```python
from build123d import *

# Parameters (mm, degrees)
SKETCH1_R           = 9.5
SKETCH1_R_2         = 1.75
SKETCH1_R_3         = 2.6
SKETCH1_R_4         = 3.7
SKETCH1_R_5         = 1.6
SKETCH1_R_6         = 1.55
BOSS_EXTRUDE1_DEPTH = 3.175
FILLET1_R           = 5
FILLET2_R           = 2
BOSS_EXTRUDE2_DEPTH = 3.175
FILLET3_R           = 2
FILLET4_R           = 2
BOSS_EXTRUDE3_START = -3.175
SKETCH4_R           = 2.6
BOSS_EXTRUDE3_DEPTH = 3.175
FILLET5_R           = 5


with BuildPart() as part:
    # Sketch1 → Boss-Extrude1 (new body)
    with BuildSketch(Plane(origin=(0, 0, 0), x_dir=(1, 0, 0), z_dir=(0, 1, 0))):
        with BuildLine():
            Line((-20, -12.068401935), (-7.259795863, 5.319338683))
            ThreePointArc((-7.259795863, 5.319338683), (0, 9), (7.259795863, 5.319338683))
            Line((7.259795863, 5.319338683), (20, -12.068401935))
            Line((20, -12.068401935), (20, -27.9))
            Line((20, -27.9), (31.6, -27.9))
            Line((31.6, -27.9), (31.6, -42.165352614))
            ThreePointArc((31.6, -42.165352614), (51.458612907, -58.2971553), (34, -77))
            Line((34, -77), (23.797619048, -77))
            Line((23.797619048, -77), (20, -93.5))
            Line((20, -93.5), (-20, -93.5))
            Line((-20, -93.5), (-31.6, -43.1))
            Line((-31.6, -43.1), (-31.6, -27.9))
            Line((-31.6, -27.9), (-20, -27.9))
            Line((-20, -27.9), (-20, -12.068401935))
        make_face()
        with Locations(Location((34, -59.5, 0), (0, 0, 270))):
            Circle(SKETCH1_R, mode=Mode.SUBTRACT)
        with Locations(Location((28.294653467, -47.264844875, 0), (0, 0, 270))):
            Circle(SKETCH1_R_2, mode=Mode.SUBTRACT)
        with Locations(Location((39.705346533, -71.735155125, 0), (0, 0, 270))):
            Circle(SKETCH1_R_2, mode=Mode.SUBTRACT)
        with Locations(Location((-24, -35.5, 0), (0, 0, 270))):
            Circle(SKETCH1_R_3, mode=Mode.SUBTRACT)
        with Locations(Location((24, -35.5, 0), (0, 0, 270))):
            Circle(SKETCH1_R_3, mode=Mode.SUBTRACT)
        with Locations(Location((0, 0, 0), (0, 0, 270))):
            Circle(SKETCH1_R_4, mode=Mode.SUBTRACT)
        with Locations(Location((-12.5, -39.3, 0), (0, 0, 270))):
            Circle(SKETCH1_R_5, mode=Mode.SUBTRACT)
        with Locations(Location((-6.75, -19.3, 0), (0, 0, 270))):
            Circle(SKETCH1_R_6, mode=Mode.SUBTRACT)
        with Locations(Location((6.75, -19.3, 0), (0, 0, 270))):
            Circle(SKETCH1_R_6, mode=Mode.SUBTRACT)
        with Locations(Location((7.5, -39.3, 0), (0, 0, 90))):
            Circle(SKETCH1_R_5, mode=Mode.SUBTRACT)
        with Locations(Location((7.5, -88.2, 0), (0, 0, 270))):
            Circle(SKETCH1_R_5, mode=Mode.SUBTRACT)
        with Locations(Location((-12.5, -88.2, 0), (0, 0, 90))):
            Circle(SKETCH1_R_5, mode=Mode.SUBTRACT)
        with BuildLine():
            Line((0, -53.5), (-1.291796068, -53.5))
            ThreePointArc((-1.291796068, -53.5), (-17, -59.5), (-1.291796068, -65.5))
            Line((-1.291796068, -65.5), (0, -65.5))
            ThreePointArc((0, -65.5), (6, -59.5), (0, -53.5))
        make_face(mode=Mode.SUBTRACT)
    extrude(amount=BOSS_EXTRUDE1_DEPTH)

    # Fillet1
    fillet1_edges = [part.edges().sort_by_distance(p)[0] for p in [
        (-31.6, 1.5875, 43.1),
        (-31.6, 1.5875, 27.9),
        (-20, 1.5875, 27.9),
        (-20, 1.5875, 12.068401935),
        (20, 1.5875, 12.068401935),
        (20, 1.5875, 27.9),
        (31.6, 1.5875, 27.9),
        (31.6, 1.5875, 42.165352614),
        (23.797619048, 1.5875, 77),
    ]]
    fillet(fillet1_edges, radius=FILLET1_R)

    # Fillet2
    fillet2_edges = [part.edges().sort_by_distance(p)[0] for p in [
        (-20, 1.5875, 93.5),
        (20, 1.5875, 93.5),
    ]]
    fillet(fillet2_edges, radius=FILLET2_R)

    # Sketch3 → Boss-Extrude2 (add)
    with BuildSketch(Plane(origin=(0, 3.175, 0), x_dir=(1, 0, 0), z_dir=(0, 1, 0))):
        Polygon((21.631006471, -86.413558093), (31.631006471, -86.413558093), (31.631006471, -81), (37.631006471, -81), (37.631006471, -92.413558093), (20.25005409, -92.413558093), align=None)
    extrude(amount=-BOSS_EXTRUDE2_DEPTH)

    # Fillet3
    fillet3_edges = [part.edges().sort_by_distance(p)[0] for p in [
        (21.631006471, 1.5875, 86.413558093),
        (31.631006471, 1.5875, 86.413558093),
        (31.631006471, 1.5875, 81),
        (37.631006471, 1.5875, 81),
        (37.631006471, 1.5875, 92.413558093),
    ]]
    fillet(fillet3_edges, radius=FILLET3_R)

    # Fillet4
    # the kernel refuses this fillet: 2 mm, written as the material it adds along each edge
    with BuildSketch(Plane(origin=(20.357070738, 0, 91.948589209), x_dir=(-0.22429460454884337, 0, 0.974521385281143), z_dir=(0, 1, 0))) as fillet4_piece_1:
        with BuildLine():
            CenterArc((1.551860901, 1.686696047), FILLET4_R, 237.495369906, 9.676681216)
            ThreePointArc((0.77593045, -0.156651976), (0.395792845, -0.039554126), (0, 0))
            Line((0, 0), (0.477125378, 0))
        make_face()
    extrude(amount=3.175)
    # the kernel refuses this fillet: 2 mm, written as the material it adds along each edge
    with BuildSketch(Plane(origin=(20.25005409, 3.175, 92.413558093), x_dir=(1, 0, 0), z_dir=(0, -1, 0))) as fillet4_2_piece_1:
        with BuildLine():
            CenterArc((0.898626945, 2), FILLET4_R, 226.75155148, 43.24844852)
            Line((-0.471699589, 0.543220953), (-0.608732242, 0.397543049))
            ThreePointArc((-0.608732242, 0.397543049), (-0.381915572, 0.139094357), (-0.140266399, -0.142566957))
            Line((-0.140266399, -0.142566957), (0, -0.2))
            Line((0, -0.2), (0.898626945, -0.2))
            Line((0.898626945, -0.2), (0.898626945, 0))
        make_face()
    extrude(amount=3.175)

    # Sketch4 → Boss-Extrude3 (add)
    with BuildSketch(Plane(origin=(0, 3.175, 0), x_dir=(1, 0, 0), z_dir=(0, 1, 0)).offset(BOSS_EXTRUDE3_START)):
        with BuildLine():
            Line((13.146507893, -2.714804316), (7.259795863, 5.319338683))
            ThreePointArc((7.259795863, 5.319338683), (0, 9), (-7.259795863, 5.319338683))
            Line((-7.259795863, 5.319338683), (-13.146507893, -2.714804316))
            Line((-13.146507893, -2.714804316), (-20, 2.306830778))
            Line((-20, 2.306830778), (-20, 25))
            Line((-20, 25), (20, 25))
            Line((20, 25), (20, 2.306830778))
            Line((20, 2.306830778), (13.146507893, -2.714804316))
        make_face()
        with Locations(Location((-15, 20, 0), (0, 0, 270))):
            Circle(SKETCH4_R, mode=Mode.SUBTRACT)
        with Locations(Location((15, 20, 0), (0, 0, 270))):
            Circle(SKETCH4_R, mode=Mode.SUBTRACT)
    extrude(amount=BOSS_EXTRUDE3_DEPTH)

    # Fillet5
    fillet5_edges = [part.edges().sort_by_distance(p)[0] for p in [
        (13.146507893, 1.5875, 2.714804316),
        (20, 1.5875, -2.306830778),
        (20, 1.5875, -25),
        (-20, 1.5875, -25),
        (-20, 1.5875, -2.306830778),
        (-13.146507893, 1.5875, 2.714804316),
    ]]
    fillet(fillet5_edges, radius=FILLET5_R)


solid = part.part
```
Geometry: final body of the model. Coordinates: model frame, mm. A direction names the side the tool comes from. Round coordinates to 2 decimals unless told otherwise and drop trailing zeros. Order: outer loops, then holes, each group sorted by start corner. A loop starts at its lowest first (then second) coordinate and runs counter-clockwise, first axis right, second up. Notation, with made-up numbers: M -34,32 L 4,32 A32 ccw 4,61 Z; hole C 32,-19.75 d2. An arc over 180 degrees is marked long. Use one line per item in the form item = value. Start each with the question number.
Q1. Material intervals for line 1 (X direction, y = 1.2, z = 35.5); line 2 (Z direction, x = 30.5, y = 2.15); line 3 (X direction, y = 0.8, z = 88.2), sorted ascending. Write a range as [from, to].
Q2. Cut plane D-D (y = 1.1). Count the separate pieces of the cut face and the enclosed holes in it, and give its area (3 significant figures).
Q3. Cut plane A-A (z = 19.3). Return loops of the section in (x, y) (3 decimals), and give its area (3 significant figures).
Q4. Cut plane B-B (z = 35.5). Return loops of the section in (x, y) (3 decimals).
Q5. Mould query, pull axis Z, two halves, no side actions, for faces 5 (the face through (37.997, 1.565, 71.356)), 6 (the face through (36.854, 1.565, 68.561)), 7 (the face through (32.8, 1.6, 40.4)), 8 (the face through (-25.837, 1.565, 68.139)). Classes: +Z half, -Z half, draft (parallel to the pull), parting line (faces both ways), or undercut.
Q6. Pin query (flat end, axial travel): pin 1 Ø4.5 at (x, z) = (0, 0) entering from -Y; pin 2 Ø1.8 at (x, y) = (26, 1.5) entering from -Z; pin 3 Ø1.5 at (y, z) = (2.5, 71) entering from +X; pin 4 Ø1.6 at (x, y) = (31.5, 1) entering from +Z. Return the tip coordinate at first contact, or that it passes through.
Q7. Cut plane C-C (x = 46.5). Return loops of the section in (y, z) (3 decimals).
Q8. Access query for faces 1 (the face through (22.555, 1.565, 82.4)), 2 (the face through (-21.43, 1.61, 26.4)), 3 (the face through (-17.59, 1.57, 8.78)), 4 (the face through (19.745, 1.61, 12.128)). Directions: +Z, -Z, +X, -X, +Y, -Y. A direction counts if a zero-diameter tool reaches every point of the face in a straight line with its end or side. Return the directions, or none.
Geometry results:
q1.line_1 = [-31.6, -26.6], [-21.4, 21.4], [26.6, 31.6]
q1.line_2 = [29.77, 50.67], [68.33, 77], [86.21, 92.41]
q1.line_3 = [-21.22, -14.1], [-10.9, 5.9], [9.1, 37.63]
q2.separate_pieces = 1
q2.enclosed_holes = 15
q2.area = 5,630 mm^2
q3.outline = M -20,0 L -8.3,0 L -8.3,3.175 L -20,3.175 Z; M -5.2,0 L 5.2,0 L 5.2,3.175 L -5.2,3.175 Z; M 8.3,0 L 20,0 L 20,3.175 L 8.3,3.175 Z
q3.area = 107 mm^2
q4.outline = M -31.6,0 L -26.6,0 L -26.6,3.175 L -31.6,3.175 Z; M -21.4,0 L 21.4,0 L 21.4,3.175 L -21.4,3.175 Z; M 26.6,0 L 31.6,0 L 31.6,3.175 L 26.6,3.175 Z
q5.face_5 = undercut
q5.face_6 = undercut
q5.face_7 = -Z half
q5.face_8 = +Z half
q6.pin_1 = through
q6.pin_2 = 27.9
q6.pin_3 = 47.81
q6.pin_4 = 92.41
q7.outline = M 0,47.253 L 3.175,47.253 L 3.175,71.747 L 0,71.747 Z
q8.face_1 = +Y, -Y
q8.face_2 = -Z, -X, +Y, -Y
q8.face_3 = -X, +Y, -Y
q8.face_4 = +X, +Y, -Y
